from build123d import *

# Parameters (mm, degrees)
ESBO_O1_W                                            = 400
ESBO_O1_H                                            = 240
RESSALTO_EXTRUS_O1_DEPTH                             = 35
ESBO_O2_R                                            = 35
CORTE_EXTRUS_O1_DEPTH                                = 315.364438192
FURO_ROSCADO_DE_M101_D                               = 8.5
FURO_ROSCADO_DE_M101_DEPTH                           = 27.5
FURO_ROSCADO_DE_M101_TIP                             = 2.553657631
FUROS_GUIA_COM_10_0MM1_D                             = 10
FUROS_GUIA_COM_10_0MM1_DEPTH                         = 27.5
FUROS_GUIA_COM_10_0MM1_TIP                           = 3.004303095
REBAIXO_PARA_PARAFUSO_ALLEN_SEXTAVADO_DE_D           = 11
REBAIXO_PARA_PARAFUSO_ALLEN_SEXTAVADO_DE_CBORE_D     = 18
REBAIXO_PARA_PARAFUSO_ALLEN_SEXTAVADO_DE_CBORE_DEPTH = 15
FUROS_GUIA_COM_10_0MM2_D                             = 10
FURO_DE_DI_METRO_11_0_11_1_D                         = 11
FURO_DE_DI_METRO_11_0_11_1_DEPTH                     = 15
FURO_DE_DI_METRO_11_0_11_1_TIP                       = 3.304733405


with BuildPart() as part:
    # Esboço1 → Ressalto-extrusão1 (new body)
    with BuildSketch(Plane.XY):
        with Locations((0, -120)):
            Rectangle(ESBO_O1_W, ESBO_O1_H)
    extrude(amount=RESSALTO_EXTRUS_O1_DEPTH)

    # Esboço2 → Corte-extrusão1 (cut, through all)
    with BuildSketch(Plane(origin=(0, 0, 0), x_dir=(-1, 0, 0), z_dir=(0, 0, -1))):
        with Locations((0, -240)):
            Circle(ESBO_O2_R)
    extrude(amount=-CORTE_EXTRUS_O1_DEPTH, mode=Mode.SUBTRACT)

    # Furo roscado de M101
    with Locations(Plane(origin=(0, -240, 0), x_dir=(-1, 0, 0), z_dir=(0, -1, 0))):
        with Locations((-180, -17.5), (-80, -17.5), (80, -17.5), (180, -17.5)):
            Hole(FURO_ROSCADO_DE_M101_D / 2, depth=FURO_ROSCADO_DE_M101_DEPTH)
            with Locations((0, 0, -(FURO_ROSCADO_DE_M101_DEPTH + FURO_ROSCADO_DE_M101_TIP / 2))):  # 118° drill point
                Cone(0, FURO_ROSCADO_DE_M101_D / 2, FURO_ROSCADO_DE_M101_TIP, mode=Mode.SUBTRACT)

    # Furos-guia com Ø10.0mm1
    with Locations(Plane(origin=(0, -240, 0), x_dir=(-1, 0, 0), z_dir=(0, -1, 0))):
        with Locations((-130, -17.5), (130, -17.5)):
            Hole(FUROS_GUIA_COM_10_0MM1_D / 2, depth=FUROS_GUIA_COM_10_0MM1_DEPTH)
            with Locations((0, 0, -(FUROS_GUIA_COM_10_0MM1_DEPTH + FUROS_GUIA_COM_10_0MM1_TIP / 2))):  # 118° drill point
                Cone(0, FUROS_GUIA_COM_10_0MM1_D / 2, FUROS_GUIA_COM_10_0MM1_TIP, mode=Mode.SUBTRACT)

    # Rebaixo para parafuso Allen sextavado de M101 (through all)
    with Locations(Plane.XY.offset(35)):
        with Locations((180, -17.5), (90, -17.5), (0, -17.5), (-90, -17.5), (-180, -17.5)):
            CounterBoreHole(REBAIXO_PARA_PARAFUSO_ALLEN_SEXTAVADO_DE_D / 2, REBAIXO_PARA_PARAFUSO_ALLEN_SEXTAVADO_DE_CBORE_D / 2, REBAIXO_PARA_PARAFUSO_ALLEN_SEXTAVADO_DE_CBORE_DEPTH)

    # Furos-guia com Ø10.0mm2 (through all)
    with Locations(Plane.XY.offset(35)):
        with Locations((135, -17.5), (-135, -17.5)):
            Hole(FUROS_GUIA_COM_10_0MM2_D / 2)

    # Furo de diâmetro Ø11.0 (11)1
    with Locations(Plane.XY.offset(35)):
        with Locations((135, -17.5), (-135, -17.5)):
            Hole(FURO_DE_DI_METRO_11_0_11_1_D / 2, depth=FURO_DE_DI_METRO_11_0_11_1_DEPTH)
            with Locations((0, 0, -(FURO_DE_DI_METRO_11_0_11_1_DEPTH + FURO_DE_DI_METRO_11_0_11_1_TIP / 2))):  # 118° drill point
                Cone(0, FURO_DE_DI_METRO_11_0_11_1_D / 2, FURO_DE_DI_METRO_11_0_11_1_TIP, mode=Mode.SUBTRACT)


solid = part.part
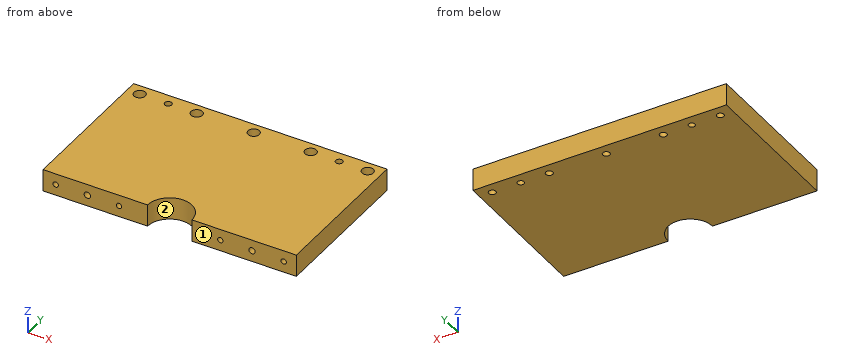
Geometry: final body of the model. Coordinates: model frame, mm. Face numbers are marked on the shaded views. Round coordinates to 2 decimals unless told otherwise and drop trailing zeros. One line per question, with ' | ' between items.
(1) Contact query for flat-ended pins moving along their axis: P1, Ø5.5, axis at x = 85.5, y = -20, coming from the +Z side; P2, Ø12, axis at x = -6, z = 25.5, coming from the -Y side. Output: stop coordinate, or through.
Check result:
P1: stops at z = 20 | P2: stops at y = -207.12
(2) Pull-direction query (X, two-part tool) for the marked faces 1 and 2; classes: +X half, -X half, draft (parallel to the pull), parting line (faces both ways), or undercut.
Check result:
face 1: draft | face 2: undercut
(3) Material intervals for line 1 along Y through (x, z) = (-180, 23.5); line 2 along Y through (x, z) = (-90, 10); line 3 along Z through (x, y) = (-180, -227), sorted ascending. Write a range as from..to.
Check result:
line 1: y = -240..-26.5, -8.5..0 | line 2: y = -240..-23, -12..0 | line 3: z = 0..13.25, 21.75..35
(4) Cut plane A-A on y = -17.5. Give the number of separate pieces and of enclosed holes in the cut face, plus the area to 3 significant figures.
Check result:
separate pieces: 8 | enclosed holes: 0 | area: 10,800 mm2
